```python
from build123d import *

# Parameters (mm, degrees)
EXTRUDE1_DEPTH       = 3.175
EXTRUDE2_DEPTH       = 6.35
EXTRUDE3_DEPTH       = 6.35
FILLET1_R            = 9.525
FILLET2_R            = 3.175
FILLET1_OF_MIRROR1_R = 9.525
FILLET2_OF_MIRROR1_R = 3.175


with BuildPart() as part:
    # Sketch1 → Extrude1 (new body, symmetric)
    with BuildSketch(Plane.XY):
        with BuildLine():
            Line((218.47175, -3.175), (186.72175, -3.175))
            ThreePointArc((186.72175, -3.175), (108.839, -28.738144468), (30.95625, -3.175))
            Line((30.95625, -3.175), (-0.79375, -3.175))
            ThreePointArc((-0.79375, -3.175), (108.839, -49.714619652), (218.47175, -3.175))
        make_face()
    extrude(amount=EXTRUDE1_DEPTH, both=True)

    # Sketch2 → Extrude2 (add)
    with BuildSketch(Plane(origin=(0, 0, -3.175), x_dir=(-1, 0, 0), z_dir=(0, 0, -1))):
        with BuildLine():
            Line((16.5735, -77.7875), (-29.946040711, -77.7875))
            Line((-29.946040711, -77.7875), (-58.727389514, -41.240247997))
            ThreePointArc((-58.727389514, -41.240247997), (-52.51922119, -38.926209978), (-46.417495888, -36.344529471))
            Line((-46.417495888, -36.344529471), (-23.782101567, -65.0875))
            Line((-23.782101567, -65.0875), (16.5735, -65.0875))
            Line((16.5735, -65.0875), (16.5735, -77.7875))
        make_face()
    extrude2 = extrude(amount=-EXTRUDE2_DEPTH)

    # Sketch3 → Extrude3 (add)
    with BuildSketch(Plane.XY.offset(3.175)):
        with BuildLine():
            Line((179.598329003, -32.291941299), (235.1405, -3.175))
            Line((235.1405, -3.175), (218.47175, -3.175))
            ThreePointArc((218.47175, -3.175), (200.202420522, -19.2920167), (179.598329003, -32.291941299))
        make_face()
    extrude3 = extrude(amount=-EXTRUDE3_DEPTH)

    # Fillet1
    fillet1_edges = [part.edges().sort_by_distance(p)[0] for p in [
        (29.946040711, -77.7875, 0),
        (58.727389514, -41.240247997, 0),
        (46.417495888, -36.344529471, 0),
        (23.782101567, -65.0875, 0),
    ]]
    fillet(fillet1_edges, radius=FILLET1_R)

    # Fillet2
    fillet2_edges = [part.edges().sort_by_distance(p)[0] for p in [
        (-16.5735, -65.0875, 0),
        (-16.5735, -77.7875, 0),
    ]]
    fillet(fillet2_edges, radius=FILLET2_R)

    # Mirror1: Extrude2, Extrude3 across plane
    add(extrude2.mirror(Plane(origin=(108.839, 0, 0), x_dir=(0, 0, 1), z_dir=(1, 0, 0))))
    add(extrude3.mirror(Plane(origin=(108.839, 0, 0), x_dir=(0, 0, 1), z_dir=(1, 0, 0))))

    # Fillet1 of Mirror1
    fillet1_of_mirror1_edges = [part.edges().sort_by_distance(p)[0] for p in [
        (187.731959289, -77.7875, 0),
        (158.950610486, -41.240247997, 0),
        (171.260504112, -36.344529471, 0),
        (193.895898433, -65.0875, 0),
    ]]
    fillet(fillet1_of_mirror1_edges, radius=FILLET1_OF_MIRROR1_R)

    # Fillet2 of Mirror1
    fillet2_of_mirror1_edges = [part.edges().sort_by_distance(p)[0] for p in [
        (234.2515, -65.0875, 0),
        (234.2515, -77.7875, 0),
    ]]
    fillet(fillet2_of_mirror1_edges, radius=FILLET2_OF_MIRROR1_R)


solid = part.part
```
Part model, mm, in its own coordinate system. A direction names the side the tool comes from. Coordinates: 2 decimals unless noted, no trailing zeros. Order: outer loops, then holes, each group sorted by start corner. A loop starts at its lowest first (then second) coordinate and runs counter-clockwise, first axis right, second up. Notation, with made-up numbers: (29, 32.5) - (35, 32.5) arc R26 ccw to (35, 60.5) - close; hole circle Ø10 at (13, 83). An arc over 180 degrees is marked (long way). Return JSON: item names as keys, results as strings. Group by question number.
Item 1: Cut at C-C (x = 78). List the corners of the cut face in (y, z) (3 decimals), plus the area to 3 significant figures.
Item 2: Pull direction Y, two halves, no side cores. Call faces 1 (the face through (109, -35, 3.175)), 2 (the face through (215, -65.088, 0)), 3 (the face through (108.214, -49.713, 0.044)): pulls with the +Y half, pulls with the -Y half, needs draft (parallel to the pull), parting line crosses it, or undercut.
Item 3: Cut at B-B (x = 206). List the corners of the cut face in (y, z) (1 decimal), plus the area to 3 significant figures.
Item 4: Which spindle directions (+Z, -Z, +X, -X, +Y, -Y) get a long thin tool onto all of the face, cutting with end or side? Do faces 4 (the face through (23.26, -64.16, 0.04)), 5 (the face through (194.3, -64.1, 0)), 6 (the face through (174.12, -60.5, -0.04)). Say none if no direction does.
Item 5: Drill centre lines: probe 1 along Y at (x, z) = (107, -1.5); probe 2 along X at (y, z) = (-54, 1.5); probe 3 along Y at (x, z) = (185, 2). Where is each one in solid material? Low to high. Write a range as from..to.
Item 6: Cut at A-A (x = 10.5). List the corners of the cut face in (y, z) (1 decimal).
Item 7: Pin check, flat tips, straight feed: pin 1 (2 mm diameter, centred on y = -70, z = 0, fed in from +X); pin 2 (2 mm diameter, centred on y = -40, z = 2, fed in from -X). Stop position of each tip, or through.
Item 8: Cut at D-D (x = 132.5). List the corners of the cut face in (y, z) (3 decimals), plus the area to 3 significant figures.
Check values:
{
 "1": {"outline": "(-46.562, -3.175) - (-25.069, -3.175) - (-25.069, 3.175) - (-46.562, 3.175) - close", "area": "136 mm2"},
 "2": {"face 1": "needs draft", "face 2": "undercut", "face 3": "pulls with the -Y half"},
 "3": {"outline": "(-77.8, -3.2) - (-65.1, -3.2) - (-65.1, 3.2) - (-77.8, 3.2) - close; (-18.5, -3.2) - (-3.2, -3.2) - (-3.2, 3.2) - (-18.5, 3.2) - close", "area": "178 mm2"},
 "4": {"face 4": "+Z, -Z, -X", "face 5": "+Z, -Z, +X", "face 6": "+Z, -Z, -Y"},
 "5": {"probe 1": "y = -49.7..-28.73", "probe 2": "x = 32.51..48.68, 169..185.16", "probe 3": "y = -74.31..-53.79, -29.46..-4.42"},
 "6": {"outline": "(-77.8, -3.2) - (-65.1, -3.2) - (-65.1, 3.2) - (-77.8, 3.2) - close; (-17.8, -3.2) - (-3.2, -3.2) - (-3.2, 3.2) - (-17.8, 3.2) - close"},
 "7": {"pin 1": "stops at x = 234.25", "pin 2": "stops at x = 41.11"},
 "8": {"outline": "(-47.867, -3.175) - (-26.591, -3.175) - (-26.591, 3.175) - (-47.867, 3.175) - close", "area": "135 mm2"}
}
